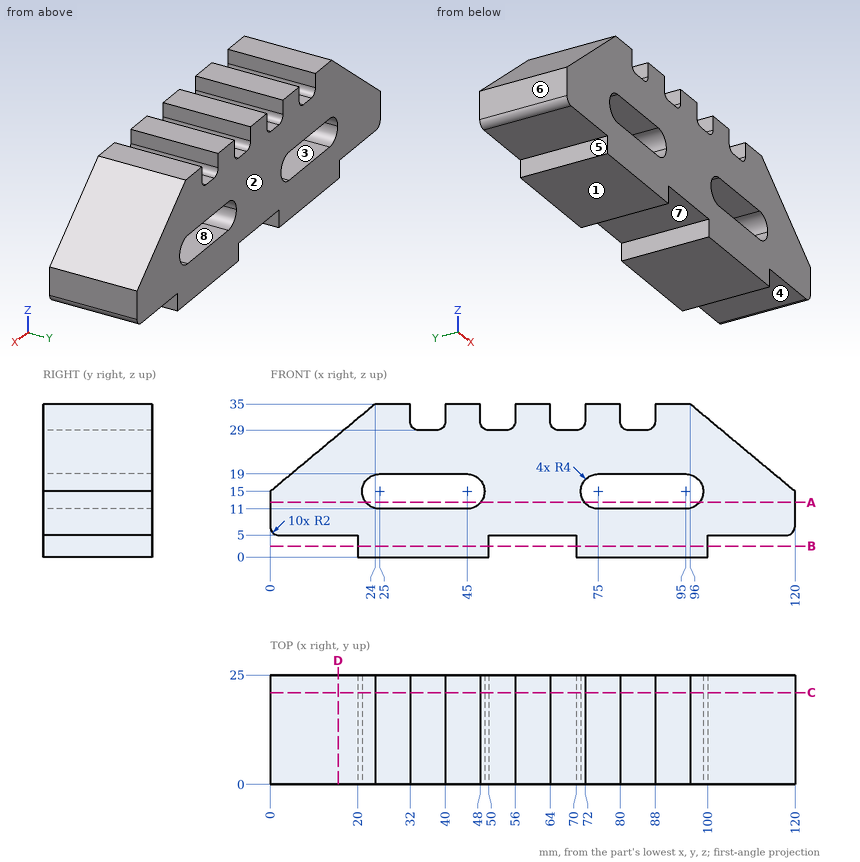
Drawing for the job (mm, zero at the part's lowest x, y, z). A direction names the side the tool comes from. Coordinates: 2 decimals unless noted, no trailing zeros. Order: outer loops, then holes, each group sorted by start corner. A loop starts at its lowest first (then second) coordinate and runs counter-clockwise, first axis right, second up. Notation, with made-up numbers: (10, 33.25) -> (34, 33.25) arc R22 cw to (34, 43.25) -> close; hole circle Ø10 at (44.25, 6.5). An arc over 180 degrees is marked (long way). Answer in a Markdown table with one row per item.
1) Which spindle directions (+Z, -Z, +X, -X, +Y, -Y) get a long thin tool onto all of the face, cutting with end or side? Do the marked faces 4, 5, 6, 7 and 8. Say none if no direction does.
Check values:
| item | result |
|---|---|
| face 4 | -Z, +X, +Y, -Y |
| face 5 | -Z, -X, +Y, -Y |
| face 6 | +Z, -Z, -X, +Y, -Y |
| face 7 | -Z, +Y, -Y |
| face 8 | +Y, -Y |
2) Band-saw the part on A-A (z = 12.5). List the corners of the cut face in (x, y), and give its area (3 significant figures).
Check values:
| item | result |
|---|---|
| outline | (0, 0) -> (21.88, 0) -> (21.88, 25) -> (0, 25) -> close; (48.12, 0) -> (71.88, 0) -> (71.88, 25) -> (48.12, 25) -> close; (98.12, 0) -> (120, 0) -> (120, 25) -> (98.12, 25) -> close |
| area | 1,690 mm2 |
3) Mould opens along Z. For the marked faces 1, 2 and 3 say: pulls with the +Z half, pulls with the -Z half, needs draft (parallel to the pull), parting line crosses it, or undercut.
Check values:
| item | result |
|---|---|
| face 1 | pulls with the -Z half |
| face 2 | needs draft |
| face 3 | undercut |
4) Drill centre lines: line 1 (X direction, y = 24, z = 15); line 2 (Z direction, x = 79, y = 8.5); line 3 (X direction, y = 22.5, z = 29.5). Where is each one in solid material? Low to high.
Check values:
| item | result |
|---|---|
| line 1 | 0 to 21, 49 to 71, 99 to 120 |
| line 2 | 0 to 11, 19 to 35 |
| line 3 | 17.4 to 32.68, 39.32 to 48.68, 55.32 to 64.68, 71.32 to 80.68, 87.32 to 102.6 |
5) Flat gauge pins, fed straight in: P1, Ø4.5, axis at y = 11.5, z = 33.5, coming from the -X side; P2, Ø4, axis at y = 12, z = 1.5, coming from the -X side; P3, Ø4.5, axis at y = 18, z = 33, coming from the +X side. Where does each tip first touch, or does it go through?
Check values:
| item | result |
|---|---|
| P1 | x = 19.5 |
| P2 | x = 20 |
| P3 | x = 101.1 |
6) Band-saw the part on B-B (z = 2.5). List the corners of the cut face in (x, y).
Check values:
| item | result |
|---|---|
| outline | (20, 0) -> (50, 0) -> (50, 25) -> (20, 25) -> close; (70, 0) -> (100, 0) -> (100, 25) -> (70, 25) -> close |
7) Band-saw the part on D-D (x = 15.5). List the corners of the cut face in (y, z).
Check values:
| item | result |
|---|---|
| outline | (0, 5) -> (25, 5) -> (25, 27.92) -> (0, 27.92) -> close |
8) Band-saw the part on C-C (y = 21). Give the number of separate pieces and of enclosed holes in the cut face, and give its area (3 significant figures).
Check values:
| item | result |
|---|---|
| separate pieces | 1 |
| enclosed holes | 2 |
| area | 2,810 mm2 |
